Autodesk Inventor part; units mm, degrees
ref_plane "YZ Plane" through (0, 0, 0) normal (1, 0, 0) x (0, 1, 0)
ref_plane "XZ Plane" through (0, 0, 0) normal (0, 1, 0) x (-1, 0, 0)
ref_plane "XY Plane" through (0, 0, 0) normal (0, 0, 1) x (1, 0, 0)
sketch "Sketch1" plane through (0, 0, 0) normal (0, 0, 1) x (1, 0, 0)
  line L0 (0, 0) -> (900, 0)
  line L1 (900, 0) -> (900, 450)
  line L2 (900, 450) -> (0, 450)
  line L3 (0, 450) -> (0, 0)
  line L4 (3, 447) -> (897, 447)
  line L5 (897, 447) -> (897, 3)
  line L6 (897, 3) -> (3, 3)
  line L7 (3, 3) -> (3, 447)
  dimension "d8" = 900
  dimension "d9" = 450
  dimension "d10" = 3
extrude "Extrusion2" add sketch "Sketch1" against normal blind 40
extrude "Extrusion3" add sketch "Sketch1" against normal blind 3 contours L3 L2 L1 L0 | L4 L5 L6 L7
sketch "Sketch2" plane through (0, 450, -40) normal (0, 1, 0) x (1, 0, 0)
  line L0 (0, -40) -> (0, 0)
  line L1 (900, -40) -> (0, -40)
  line L2 (900, -40) -> (900, 0)
  point P0 (15, -25)
  point P1 (885, -25)
  dimension "d22" = 15
  dimension "d23" = 15
  dimension "d24" = 15
  dimension "d25" = 15
hole "Hole1" at (15, 450, -15) at (885, 450, -15) direction (0, -1, 0) diameter 3.81 end through all
sketch "Sketch3" plane through (0, 0, -40) normal (-1, 0, 0) x (0, 0, 1)
  line L0 (40, 450) -> (40, 0)
  line L1 (40, 0) -> (0, 0)
  line L2 (40, 450) -> (0, 450)
  point P0 (25, 15)
  point P1 (25, 435)
  dimension "d26" = 15
  dimension "d27" = 15
  dimension "d28" = 15
  dimension "d29" = 15
hole "Hole2" at (0, 15, -15) at (0, 435, -15) direction (1, 0, 0) diameter 3.81 end through all
equation "\"d8\" = Width"
equation "\"d9\" = Depth"
equation "\"d10\" = Thickness"
equation "\"d11\" = Height"
equation "\"d13\" = Thickness"
equation "\"Width\" = 900"
equation "\"Thickness\" = 3"
equation "\"Depth\" = 450"
equation "\"Height\" = 40"
equation "\"HoleDistance\" = 15"
properties part number "shelf90"
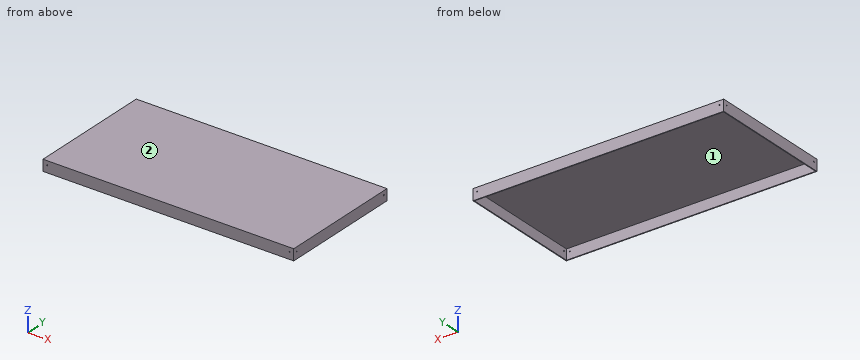
Design review of the part built by this model. Coordinates are the model's own, in mm. Face numbers are marked on the shaded views. Round coordinates to 2 decimals unless told otherwise and drop trailing zeros. Write each loop counter-clockwise with the first axis right and the second up, starting at its lowest first coordinate (ties: lowest second). Pieces come first, ordered by that corner, then holes. Notation, with made-up numbers: (-17.75, 76.5) -> (14.25, 76.5) arc R12 ccw to (14.25, 97.5) -> close; hole circle Ø2 at (79.5, 30). An arc over 180 degrees is marked (long way). Write item = value, one per line. Start each with the question number.
1) Clearance check with a flat-ended pin moving along its axis: pin 1 (3 mm diameter, centred on x = 15, z = -15, fed in from +Y). State where the tip first meets the part, or that it passes through.
2) Mouldability with a two-part tool opening along X and no side actions: class the marked faces 1 and 2 as +X half, -X half, draft (parallel to the pull), parting line (faces both ways), or undercut.
3) Take a section at A-A, the plane y = 29. State the section outline as (x, z) points, plus the area to 3 significant figures.
4) Wall thickness on probe 1 along X at (y, z) = (448, -15) (3 decimals); probe 2 along Y at (x, z) = (898, -15) (3 decimals); probe 3 along Y at (x, z) = (417, -17): over which ranges is each line inside the solid? List them lowest first. Write a range as from..to.
5) Take a section at C-C, the plane x = 449. State the section outline as (y, z) points, plus the area to 3 significant figures.
6) Take a section at B-B, the plane z = -30. State the section outline as (x, y) points, plus the area to 3 significant figures.
Results list:
q1.pin_1 = through
q2.face_1 = undercut
q2.face_2 = draft
q3.outline = (0, -40) -> (3, -40) -> (3, -3) -> (897, -3) -> (897, -40) -> (900, -40) -> (900, 0) -> (0, 0) -> close
q3.area = 2,920 mm²
q4.probe_1 = 0..13.095, 16.905..883.095, 886.905..900
q4.probe_2 = 0..13.095, 16.905..433.095, 436.905..450
q4.probe_3 = 0..3, 447..450
q5.outline = (0, -40) -> (3, -40) -> (3, -3) -> (447, -3) -> (447, -40) -> (450, -40) -> (450, 0) -> (0, 0) -> close
q5.area = 1,570 mm²
q6.outline = (0, 0) -> (900, 0) -> (900, 450) -> (0, 450) -> close; hole (3, 3) -> (897, 3) -> (897, 447) -> (3, 447) -> close
q6.area = 8,060 mm²
